```python
from build123d import *

# Parameters (mm, degrees)
SKETCH1_W           = 10.16
SKETCH1_H           = 10.16
BOSS_EXTRUDE1_DEPTH = 3.81
SKETCH2_R           = 1.524
CUT_EXTRUDE1_DEPTH  = 3.81
SKETCH3_R           = 1.01473
CUT_EXTRUDE3_DEPTH  = 10.16


with BuildPart() as part:
    # Sketch1 → Boss-Extrude1 (new body)
    with BuildSketch(Plane.XY):
        Rectangle(SKETCH1_W, SKETCH1_H)
    extrude(amount=BOSS_EXTRUDE1_DEPTH)

    # Sketch2 → Cut-Extrude1 (cut)
    with BuildSketch(Plane.XY.offset(3.81)):
        with Locations((2.54, 0)):
            Circle(SKETCH2_R)
        with Locations((-2.54, 0)):
            Circle(SKETCH2_R)
    extrude(amount=-CUT_EXTRUDE1_DEPTH, mode=Mode.SUBTRACT)

    # Sketch3 → Cut-Extrude3 (cut)
    with BuildSketch(Plane.XZ.offset(5.08)):
        with Locations((0, 1.016)):
            Circle(SKETCH3_R)
        with BuildLine():
            ThreePointArc((1.01473, 1.016), (0, 0.00127), (-1.01473, 1.016))
            Line((-1.01473, 1.016), (-1.01473, 0))
            Line((-1.01473, 0), (1.01473, 0))
            Line((1.01473, 0), (1.01473, 1.016))
        make_face()
    extrude(amount=-CUT_EXTRUDE3_DEPTH, mode=Mode.SUBTRACT)


solid = part.part
```
Read the model definition and answer for the solid it produces. Units are mm, in the model's axes. Give positions to 0.01 mm unless a question says otherwise; leave off trailing zeros. Write each loop counter-clockwise with the first axis right and the second up, starting at its lowest first coordinate (ties: lowest second). Pieces come first, ordered by that corner, then holes. Notation, with made-up numbers: (20, -26) - (35, -26) arc R27 cw to (35, -10) - close; hole circle Ø1 at (-10, 25). An arc over 180 degrees is marked (long way). Write item = value, one per line. Start each with the question number.
Item 1: Find section B-B (x = 2.54). Give the vertices of the cut face in (y, z).
Item 2: Find the intervals of material crossed by probe 1 along Y at (x, z) = (-2.54, 1.75); probe 2 along X at (y, z) = (-0.5, 3.1); probe 3 along X at (y, z) = (1, 1.7), in increasing order. Write a range as [from, to].
Item 3: Find section D-D (z = 3.3). Give the vertices of the cut face in (x, y).
Item 4: The mould has two halves that part along X. Classify faces 1 (the flat face through (4.4, 0.1, 0)), 2 (the flat face through (5.08, 0, 2)), 3 (the cylindrical face through (-4.063, 0.067, 1.932)): +X half, -X half, draft (parallel to the pull), parting line (faces both ways), or undercut.
Item 5: Find section A-A (z = 0.7). Give the vertices of the cut face in (x, y), then the cut area to 3 significant figures.
Item 6: Find section C-C (y = 0). State how many separate pieces and enclosed holes the cut face has, then the cut area to 3 significant figures.
Response:
q1.outline = (-5.08, 0) - (-1.52, 0) - (-1.52, 3.81) - (-5.08, 3.81) - close; (1.52, 0) - (5.08, 0) - (5.08, 3.81) - (1.52, 3.81) - close
q2.probe_1 = [-5.08, -1.52], [1.52, 5.08]
q2.probe_2 = [-5.08, -3.98], [-1.1, 1.1], [3.98, 5.08]
q2.probe_3 = [-5.08, -3.69], [-1.39, -0.75], [0.75, 1.39], [3.69, 5.08]
q3.outline = (-5.08, -5.08) - (5.08, -5.08) - (5.08, 5.08) - (-5.08, 5.08) - close; hole circle Ø3.05 at (-2.54, 0); hole circle Ø3.05 at (2.54, 0)
q4.face_1 = draft
q4.face_2 = +X half
q4.face_3 = undercut
q5.outline = (-5.08, -5.08) - (-1.01, -5.08) - (-1.01, 5.08) - (-5.08, 5.08) - close; (1.01, -5.08) - (5.08, -5.08) - (5.08, 5.08) - (1.01, 5.08) - close; hole circle Ø3.05 at (-2.54, 0); hole circle Ø3.05 at (2.54, 0)
q5.area = 68.0 mm²
q6.separate_pieces = 3
q6.enclosed_holes = 0
q6.area = 11.8 mm²
